Check sheet for the modelled part. Datum: model origin and axes. Units: mm. Give positions to 0.01 mm unless a question says otherwise; leave off trailing zeros. Loops run counter-clockwise (first coordinate to the right, second up) from the corner with the lowest first, then second, coordinate; pieces in that order, holes last. Notation, with made-up numbers: (-24.5, 28.25) - (-19.5, 28.25) arc R20 ccw to (-19.5, 63.25) - close; hole circle Ø7 at (28.25, -28.75). An arc over 180 degrees is marked (long way). Answer in a Markdown table with one row per item. Add a question column.
(1) Go/stop test with flat-tipped pins: P1, Ø4, axis at y = 2, z = -3.5, coming from the +X side; P2, Ø1, axis at y = 6, z = -1.5, coming from the -X side; P3, Ø24, axis at x = 150, y = 0, coming from the -Z side; P4, Ø18, axis at x = -150, y = 0, coming from the -Z side. Record where each tip stops, or that it passes through.
(2) Sectioned sample at A-A on y = 0. Enter the section's corners in (x, z), then the cut area to 3 significant figures.
(3) Thickness scan on L1, parallel to X at y = -0.5, z = -3; L2, parallel to Y at x = -150, z = 1; L3, parallel to X at y = -4.5, z = -2.75. Record the ranges inside material, lowest first.
(4) Sectioned sample at B-B on z = 3.25. Enter the section's corners in (x, y).
from build123d import *

# Parameters (mm, degrees)
BOSS_EXTRUDE1_DEPTH     = 5
SKETCH2_R               = 10
SKETCH2_R_2             = 7.5
CUT_EXTRUDE1_DEPTH      = 1
CUT_EXTRUDE1_DEPTH_BACK = 11


with BuildPart() as part:
    # Sketch1 → Boss-Extrude1 (new body, symmetric)
    with BuildSketch(Plane.XY):
        with BuildLine():
            Line((-150, 20), (150, 20))
            ThreePointArc((150, 20), (170, 0), (150, -20))
            Line((150, -20), (-150, -20))
            ThreePointArc((-150, -20), (-170, 0), (-150, 20))
        make_face()
    extrude(amount=BOSS_EXTRUDE1_DEPTH, both=True)

    # Sketch2 → Cut-Extrude1 (cut, two sides)
    with BuildSketch(Plane.XY.offset(5)) as cut_extrude1_sk:
        with Locations((-150, 0)):
            Circle(SKETCH2_R)
        with Locations((150, 0)):
            Circle(SKETCH2_R_2)
    extrude(amount=CUT_EXTRUDE1_DEPTH, mode=Mode.SUBTRACT)
    extrude(cut_extrude1_sk.sketch, amount=-CUT_EXTRUDE1_DEPTH_BACK, mode=Mode.SUBTRACT)


solid = part.part
Reply:
| question | item | result |
|---|---|---|
| 1 | P1 | x = 170 |
| 1 | P2 | x = -169.23 |
| 1 | P3 | z = -5 |
| 1 | P4 | through |
| 2 | outline | (-170, -5) - (-160, -5) - (-160, 5) - (-170, 5) - close; (-140, -5) - (142.5, -5) - (142.5, 5) - (-140, 5) - close; (157.5, -5) - (170, -5) - (170, 5) - (157.5, 5) - close |
| 2 | area | 3,050 mm^2 |
| 3 | L1 | -169.99 to -159.99, -140.01 to 142.52, 157.48 to 169.99 |
| 3 | L2 | -20 to -10, 10 to 20 |
| 3 | L3 | -169.49 to -158.93, -141.07 to 144, 156 to 169.49 |
| 4 | outline | (-150, -20) - (150, -20) arc R20 ccw to (150, 20) - (-150, 20) arc R20 ccw to start; hole circle Ø20 at (-150, 0); hole circle Ø15 at (150, 0) |
